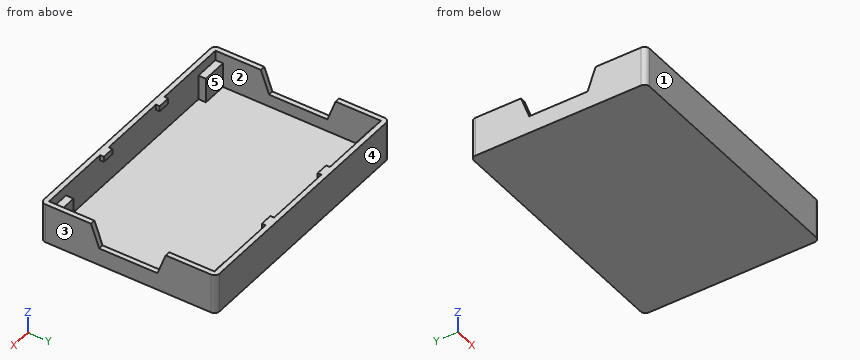
```python
from build123d import *

# Parameters (mm, degrees)
SKETCH1_W                            = 70.5
SKETCH1_H                            = 101.8
SKETCH1_W_2                          = 66.5
SKETCH1_H_2                          = 97.8
BOSS_EXTRUDE1_BOARD_4MM_DEPTH        = 4
SKETCH2_W                            = 101.8
SKETCH2_H                            = 70.5
BOSS_EXTRUDE2_UNDER_10MS_DEPTH       = 10
SKETCH3_W                            = 101.8
SKETCH3_H                            = 70.5
BOSS_EXTRUDE3_BOTTOM_COVER_2MM_DEPTH = 2
SKETCH4_W                            = 5
SKETCH4_H                            = 3.5
BOSS_EXTRUDE4_DEPTH                  = 2.2
SKETCH5_W                            = 128.386338002
SKETCH5_H                            = 30
CUT_EXTRUDE1_CUT_USB_DEPTH           = 9
CUT_EXTRUDE1_CUT_USB_DRAFT           = -20
FILLET1_R                            = 2


with BuildPart() as part:
    # Sketch1 → Boss-Extrude1-board-4mm (new body)
    with BuildSketch(Plane(origin=(0, 0, 0), x_dir=(0, 1, 0), z_dir=(0, 0, 1))):
        Rectangle(SKETCH1_W, SKETCH1_H)
        Rectangle(SKETCH1_W_2, SKETCH1_H_2, mode=Mode.SUBTRACT)
    extrude(amount=BOSS_EXTRUDE1_BOARD_4MM_DEPTH)

    # Sketch2 → Boss-Extrude2-under-10ms (add)
    with BuildSketch(Plane(origin=(0, 0, 0), x_dir=(1, 0, 0), z_dir=(0, 0, -1))):
        Rectangle(SKETCH2_W, SKETCH2_H)
        Polygon((-48.9, 30.25), (-38.9, 30.25), (-38.9, 33.25), (38.9, 33.25), (38.9, 30.25), (48.9, 30.25), (48.9, -30.25), (38.9, -30.25), (38.9, -33.25), (-38.9, -33.25), (-38.9, -30.25), (-48.9, -30.25), align=None, mode=Mode.SUBTRACT)
    extrude(amount=BOSS_EXTRUDE2_UNDER_10MS_DEPTH)

    # Sketch3 → Boss-Extrude3-bottom-cover-2mm (add)
    with BuildSketch(Plane(origin=(0, 0, -10), x_dir=(1, 0, 0), z_dir=(0, 0, -1))):
        Rectangle(SKETCH3_W, SKETCH3_H)
    extrude(amount=BOSS_EXTRUDE3_BOTTOM_COVER_2MM_DEPTH)

    # Sketch4 → Boss-Extrude4 (add)
    with BuildSketch(Plane.XY.offset(1.8)):
        with Locations((-16.4, 33.5)):
            Rectangle(SKETCH4_W, SKETCH4_H)
        with Locations((-16.4, -33.5)):
            Rectangle(SKETCH4_W, SKETCH4_H)
        with Locations((16.4, -33.5)):
            Rectangle(SKETCH4_W, SKETCH4_H)
        with Locations((16.4, 33.5)):
            Rectangle(SKETCH4_W, SKETCH4_H)
    extrude(amount=BOSS_EXTRUDE4_DEPTH)


with BuildPart() as cut_extrude1_cut_usb_tool:
    # Sketch5 → Cut-Extrude1-cut-usb (with draft: the straight prism first)
    with BuildSketch(Plane.XY.offset(4)):
        Rectangle(SKETCH5_W, SKETCH5_H)
    extrude(amount=-CUT_EXTRUDE1_CUT_USB_DEPTH)
    # Cut-Extrude1-cut-usb: the draft: its side faces are tilted about the plane it starts from
    cut_extrude1_cut_usb_sides = [cut_extrude1_cut_usb_tool.faces().sort_by_distance(p)[0] for p in [
        (0, -15, -0.5),
        (64.193169001, 0, -0.5),
        (0, 15, -0.5),
        (-64.193169001, 0, -0.5),
    ]]
    draft(cut_extrude1_cut_usb_sides, Plane.XY.offset(4), CUT_EXTRUDE1_CUT_USB_DRAFT)


with BuildPart() as part_1:
    add(part.part)

    # Cut-Extrude1-cut-usb: cut by cut_extrude1_cut_usb_tool
    add(cut_extrude1_cut_usb_tool.part, mode=Mode.SUBTRACT)

    # Fillet1
    fillet1_edges = [part_1.edges().sort_by_distance(p)[0] for p in [
        (50.9, -35.25, -4),
        (-50.9, -35.25, -4),
        (-50.9, 35.25, -4),
        (50.9, 35.25, -4),
    ]]
    fillet(fillet1_edges, radius=FILLET1_R)


solid = part_1.part
```
Here's how the part is built. I have some questions about the finished solid (model axes, mm). Face numbers are marked on the shaded views. A direction names the side the tool comes from. Coordinates: 2 decimals unless noted, no trailing zeros. Order: outer loops, then holes, each group sorted by start corner. A loop starts at its lowest first (then second) coordinate and runs counter-clockwise, first axis right, second up.
1) Imagine slicing it at A-A on z = -6.5. List the corners of the cut face in (x, y) for me.
2) Imagine slicing it at C-C on y = -21. List the corners of the cut face in (x, z) for me.
3) We'd pull the mould along X, two halves only. Please class the marked faces 1, 2 and 3: +X half, -X half, draft (parallel to the pull), parting line (faces both ways), or undercut.
4) Will these pins go through, and if not, where does the flat tip stop? pin 1 (0.9 mm diameter, centred on x = 45.5, y = 32, fed in from +Z); pin 2 (3 mm diameter, centred on x = -20, y = 4, fed in from +Z); pin 3 (0.6 mm diameter, centred on x = -50.5, y = -4.5, fed in from +Z).
5) Which directions (+Z, -Z, +X, -X, +Y, -Y) give clear straight access to the entire face, cutting with the end or side of a thin tool? Please do the marked faces 4 and 5.
6) Imagine slicing it at D-D on x = -9. List the corners of the cut face in (y, z) for me, and give its area (3 significant figures).
7) I need wall thicknesses on line 1 (Y direction, x = -41, z = 2); line 2 (X direction, y = -16.5, z = -6.5); line 3 (Y direction, x = 43, z = -2.25). Which ranges of each line are inside material? Lowest first, please.
8) Imagine slicing it at B-B on z = -1. List the corners of the cut face in (x, y) for me, and give its area (3 significant figures).
Response values:
1. outline: (-50.9, -33.25) arc R2 ccw to (-48.9, -35.25) - (48.9, -35.25) arc R2 ccw to (50.9, -33.25) - (50.9, 33.25) arc R2 ccw to (48.9, 35.25) - (-48.9, 35.25) arc R2 ccw to (-50.9, 33.25) - close; hole (-48.9, -30.25) - (-38.9, -30.25) - (-38.9, -33.25) - (38.9, -33.25) - (38.9, -30.25) - (48.9, -30.25) - (48.9, 30.25) - (38.9, 30.25) - (38.9, 33.25) - (-38.9, 33.25) - (-38.9, 30.25) - (-48.9, 30.25) - close
2. outline: (-50.9, -12) - (50.9, -12) - (50.9, 4) - (48.9, 4) - (48.9, -10) - (-48.9, -10) - (-48.9, 4) - (-50.9, 4) - close
3. face 1: draft
3. face 2: undercut
3. face 3: +X half
4. pin 1: stops at z = 0
4. pin 2: stops at z = -10
4. pin 3: stops at z = -5
5. face 4: +Z, -Z, +X, -X, +Y
5. face 5: +Z
6. outline: (-35.25, -12) - (35.25, -12) - (35.25, 4) - (33.25, 4) - (33.25, -10) - (-33.25, -10) - (-33.25, 4) - (-35.25, 4) - close
6. area: 197 mm2
7. line 1: y = -35.25 to -33.25, 33.25 to 35.25
7. line 2: x = -50.9 to -48.9, 48.9 to 50.9
7. line 3: y = -35.25 to -30.25, 30.25 to 35.25
8. outline: (-50.9, -33.25) arc R2 ccw to (-48.9, -35.25) - (48.9, -35.25) arc R2 ccw to (50.9, -33.25) - (50.9, -13.18) - (48.9, -13.18) - (48.9, -30.25) - (38.9, -30.25) - (38.9, -33.25) - (-38.9, -33.25) - (-38.9, -30.25) - (-48.9, -30.25) - (-48.9, -13.18) - (-50.9, -13.18) - close; (-50.9, 13.18) - (-48.9, 13.18) - (-48.9, 30.25) - (-38.9, 30.25) - (-38.9, 33.25) - (38.9, 33.25) - (38.9, 30.25) - (48.9, 30.25) - (48.9, 13.18) - (50.9, 13.18) - (50.9, 33.25) arc R2 ccw to (48.9, 35.25) - (-48.9, 35.25) arc R2 ccw to (-50.9, 33.25) - close
8. area: 684 mm2
